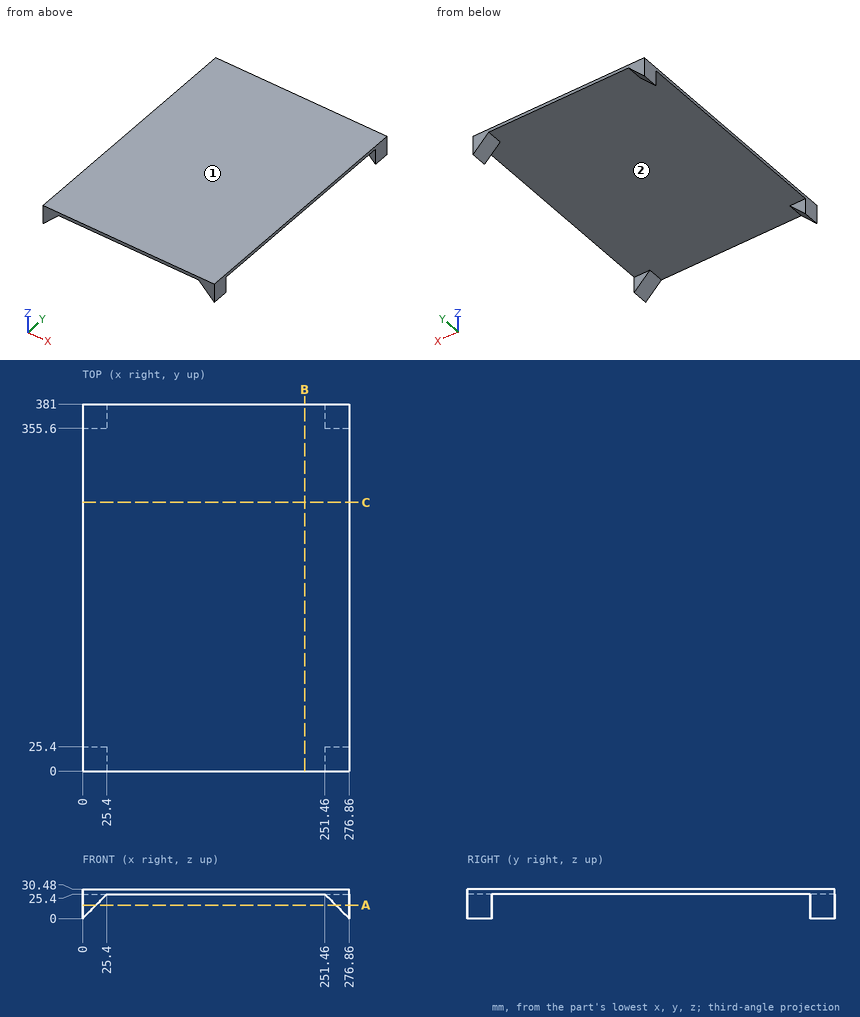
Geometry: see drawing. Coordinates: mm, zero at the bounding-box minimum. A direction names the side the tool comes from. Coordinates: 2 decimals unless noted, no trailing zeros. Loops run counter-clockwise (first coordinate to the right, second up) from the corner with the lowest first, then second, coordinate; pieces in that order, holes last. Notation, with made-up numbers: (-17, 49.5) - (0, 49.5) arc R24 ccw to (0, 68.5) - close; hole circle Ø1 at (40.25, 72). An arc over 180 degrees is marked (long way). Answer in a Markdown table with one row per item.
(1) Set-up query: the marked faces 1 and 2. Return all of +Z, -Z, +X, -X, +Y, -Y with unobstructed straight access to the full face (end or side cutting, diameter ignored); none if empty.
Model answer:
| item | result |
|---|---|
| face 1 | +Z, +X, -X, +Y, -Y |
| face 2 | -Z |
(2) Cut plane C-C on y = 279. Output: boundary loops of the cut face in (x, z).
Model answer:
| item | result |
|---|---|
| outline | (0, 25.4) - (276.86, 25.4) - (276.86, 30.48) - (0, 30.48) - close |
(3) Cut plane A-A on z = 14. Output: boundary loops of the cut face in (x, y), plus the area to 3 significant figures.
Model answer:
| item | result |
|---|---|
| outline | (0, 0) - (14, 0) - (14, 25.4) - (0, 25.4) - close; (0, 355.6) - (14, 355.6) - (14, 381) - (0, 381) - close; (262.86, 0) - (276.86, 0) - (276.86, 25.4) - (262.86, 25.4) - close; (262.86, 355.6) - (276.86, 355.6) - (276.86, 381) - (262.86, 381) - close |
| area | 1,420 mm² |
(4) Pin query (flat end, axial travel): P1, Ø3, axis at y = 243, z = 22.5, coming from the -X side. Return the tip coordinate at first contact, or that it passes through.
Model answer:
| item | result |
|---|---|
| P1 | passes through |
(5) Material intervals for L1, parallel to Z at x = 13.5, y = 71.5; L2, parallel to X at y = 362.5, z = 13.5; L3, parallel to X at y = 23, z = 8, sorted ascending. Write a range as from..to.
Model answer:
| item | result |
|---|---|
| L1 | z = 25.4..30.48 |
| L2 | x = 0..13.5, 263.36..276.86 |
| L3 | x = 0..8, 268.86..276.86 |
(6) Cut plane B-B on x = 230.5. Output: boundary loops of the cut face in (y, z).
Model answer:
| item | result |
|---|---|
| outline | (0, 25.4) - (381, 25.4) - (381, 30.48) - (0, 30.48) - close |
